```python
from build123d import *

# Parameters (mm, degrees)
SKETCH_1_W          = 86
SKETCH_1_H          = 44.4
EXTRUDE_1_DEPTH     = 19.6
EXTRUDE_2_DEPTH     = 5
SKETCH_3_W          = 40.8
SKETCH_3_H          = 42
SKETCH_3_W_2        = 41.2
CUT_EXTRUDE_1_DEPTH = 18.4
FILLET_1_R          = 3
EXTRUDE_3_DEPTH     = 0.2


with BuildPart() as part:
    # Эскиз1 → Бобышка-Вытянуть1 (new body)
    with BuildSketch(Plane.XY):
        Rectangle(SKETCH_1_W, SKETCH_1_H)
    extrude(amount=EXTRUDE_1_DEPTH)

    # Эскиз2 → Бобышка-Вытянуть2 (add)
    with BuildSketch(Plane.XY):
        with BuildLine():
            Line((43, 17.2), (43, 13.108775687))
            ThreePointArc((43, 13.108775687), (53.273546839, 0), (43, -13.108775687))
            Line((43, -13.108775687), (43, -17.2))
            ThreePointArc((43, -17.2), (57.273546839, 0), (43, 17.2))
        make_face()
    extrude(amount=EXTRUDE_2_DEPTH)

    # Эскиз3 → Вырез-Вытянуть1 (cut)
    with BuildSketch(Plane.XY.offset(19.6)):
        with Locations((-21, 0)):
            Rectangle(SKETCH_3_W, SKETCH_3_H)
        with Locations((21.2, 0)):
            Rectangle(SKETCH_3_W_2, SKETCH_3_H)
    extrude(amount=-CUT_EXTRUDE_1_DEPTH, mode=Mode.SUBTRACT)

    # Скругление1
    fillet_1_edges = [part.edges().sort_by_distance(p)[0] for p in [
        (-41.4, -21, 10.4),
        (-41.4, 21, 10.4),
        (-43, -22.2, 9.8),
        (-43, 22.2, 9.8),
    ]]
    fillet(fillet_1_edges, radius=FILLET_1_R)

    # Эскиз4 → Бобышка-Вытянуть3 (add)
    with BuildSketch(Plane(origin=(0, 0, 0), x_dir=(-1, 0, 0), z_dir=(0, 0, -1))):
        with BuildLine():
            Line((-49.811541671, 14.334875645), (-30.869317388, 22.2))
            ThreePointArc((-30.869317388, 22.2), (-45.401918337, 30.45743659), (-49.811541671, 14.334875645))
        make_face()
        with BuildLine():
            Line((43, 10.515346091), (29.589006911, 22.2))
            ThreePointArc((29.589006911, 22.2), (47.015516822, 28.662653345), (43, 10.515346091))
        make_face()
        with BuildLine():
            Line((43, -10.515346091), (29.589006911, -22.2))
            ThreePointArc((29.589006911, -22.2), (47.015516822, -28.662653345), (43, -10.515346091))
        make_face()
        with BuildLine():
            Line((-49.811541671, -14.334875645), (-30.869317388, -22.2))
            ThreePointArc((-30.869317388, -22.2), (-45.401918337, -30.45743659), (-49.811541671, -14.334875645))
        make_face()
    extrude(amount=-EXTRUDE_3_DEPTH)


solid = part.part
```
Can you work these out from the model? Positions are in its coordinate system, mm. A direction names the side the tool comes from. Give positions to 0.01 mm unless a question says otherwise; leave off trailing zeros. Loops run counter-clockwise (first coordinate to the right, second up) from the corner with the lowest first, then second, coordinate; pieces in that order, holes last. Notation, with made-up numbers: M -37.75,46.5 L -8.75,46.5 A16 cw -8.75,73.5 Z; hole C -32.75,30 d10. An arc over 180 degrees is marked long. Use one line per item in the form item = value. Start each with the question number.
(1) I want a section at D-D, the plane x = -35.5. Write out the boundary of the cut face in (y, z), and give its area (3 significant figures).
(2) I want a section at C-C, the plane z = 13. Write out the boundary of the cut face in (x, y).
(3) I want a section at A-A, the plane z = 3.25. Write out the boundary of the cut face in (x, y), and give its area (3 significant figures).
(4) I want a section at B-B, the plane y = -24. Write out the boundary of the cut face in (x, z).
(5) Thinking about a two-plate mould opening in Y: for faces 3 (the flat face through (41.8, 0, 11)), 4 (the flat face through (1, 22.2, 10)), 5 (the flat face through (3, 0, 0)), which applies, released by +Y, released by -Y, zero draft, split by the parting line, or undercut?
(6) On a 3-axis mill with a long thin cutter (end or side, diameter ignored), from which of +Z, -Z, +X, -X, +Y, -Y can I reach the whole of each face in a straight line? I mean faces 1 (the flat face through (21, 0, 1.2)), 2 (the flat face through (-42, -23, 0.2)). Say none if no direction works.
(7) I'm going to push flat-ended pins straight in: P1, Ø6, axis at y = -14, z = 10, coming from the +X side; P2, Ø6, axis at x = -34, z = 14.5, coming from the +Y side; P3, Ø6, axis at x = -19, z = 8, coming from the -Y side; P4, Ø1.5, axis at y = -23, z = 15.5, coming from the -X side. Where does each tip first touch, or does it pass through?
(8) Please list where these lines run through material, in increasing order: line 1 (X direction, y = 6.5, z = 12); line 2 (Y direction, x = -37.5, z = 3); line 3 (Y direction, x = -0.5, z = 3.75).
Worked out:
q1.outline = M -30.23,0 L 30.23,0 L 30.23,0.2 L 22.2,0.2 L 22.2,19.6 L 21,19.6 L 21,1.2 L -21,1.2 L -21,19.6 L -22.2,19.6 L -22.2,0.2 L -30.23,0.2 Z
q1.area = 101 mm²
q2.outline = M -43,-19.2 A3 ccw -40,-22.2 L 43,-22.2 L 43,22.2 L -40,22.2 A3 ccw -43,19.2 Z; hole M -41.4,-18 A3 ccw -38.4,-21 L -0.6,-21 L -0.6,21 L -38.4,21 A3 ccw -41.4,18 Z; hole M 0.6,-21 L 41.8,-21 L 41.8,21 L 0.6,21 Z
q3.outline = M -43,-19.2 A3 ccw -40,-22.2 L 43,-22.2 L 43,-17.2 A17.5 ccw 43,17.2 L 43,22.2 L -40,22.2 A3 ccw -43,19.2 Z; hole M -41.4,-18 A3 ccw -38.4,-21 L -0.6,-21 L -0.6,21 L -38.4,21 A3 ccw -41.4,18 Z; hole M 0.6,-21 L 41.8,-21 L 41.8,21 L 0.6,21 Z; hole M 43,-13.11 A13.5 ccw 43,13.11 Z
q3.area = 543 mm²
q4.outline = M -50.11,0 L -30.01,0 L -30.01,0.2 L -50.11,0.2 Z; M 31.29,0 L 51.39,0 L 51.39,0.2 L 31.29,0.2 Z
q5.face_3 = undercut
q5.face_4 = released by +Y
q5.face_5 = zero draft
q6.face_1 = +Z
q6.face_2 = +Z, -X, -Y
q7.P1 = 43
q7.P2 = 22.2
q7.P3 = -22.2
q7.P4 = through
q8.line_1 = -43 to -41.4, -0.6 to 0.6, 41.8 to 43
q8.line_2 = -22.2 to -21, 21 to 22.2
q8.line_3 = -22.2 to 22.2
